Source: CAD feature listing. Evaluate the final solid. Frame: model axes, mm. Give positions to 0.01 mm unless a question says otherwise; leave off trailing zeros. Order: outer loops, then holes, each group sorted by start corner. A loop starts at its lowest first (then second) coordinate and runs counter-clockwise, first axis right, second up. Notation, with made-up numbers: M -27,43 L 4,43 A22 cw 4,53 Z; hole C 30,36 d1. An arc over 180 degrees is marked long. One line per question, with ' | ' between items. Start each with the question number.
from build123d import *

# Parameters (mm, degrees)
SKETCH_7_R           = 35
SKETCH_7_R_2         = 15
EXTRUDE_1_DEPTH      = 15
EXTRUDE_2_REACH      = 817.889
EXTRUDE_2_END_RADIUS = 35
SKETCH_5_R           = 22.5
SKETCH_8_W           = 185.294970715
SKETCH_8_H           = 135.350234673
CUT_EXTRUDE_1_DEPTH  = 25


with BuildPart() as part:
    # 草图7 → 凸台-拉伸1 (new, symmetric)
    with BuildSketch(Plane(origin=(0, 0, 0), x_dir=(1, 0, 0), z_dir=(0, 1, 0))):
        with Locations(Location((0, -500, 0), (0, 0, 270))):
            Circle(SKETCH_7_R)
        with Locations(Location((0, -500, 0), (0, 0, 270))):
            Circle(SKETCH_7_R_2, mode=Mode.SUBTRACT)
    extrude(amount=EXTRUDE_1_DEPTH, both=True)

    # 凸台-拉伸2: up to this cylinder (the profile starts outside it)
    extrude_2_end = Plane(origin=(0, 0, 500), z_dir=(0, -1, 0)) * Cylinder(EXTRUDE_2_END_RADIUS, 1706.778, mode=Mode.PRIVATE)
    # 草图5 → 凸台-拉伸2 (add, up to the surface)
    with BuildSketch(Plane.XY.offset(-280), mode=Mode.PRIVATE) as extrude_2_sk1:
        with Locations(Location((0, 0, 0), (0, 0, 138.189685104))):
            Circle(SKETCH_5_R)
    extrude_2_tool1 = extrude(extrude_2_sk1.sketch, amount=EXTRUDE_2_REACH, mode=Mode.PRIVATE) - extrude_2_end
    add(extrude_2_tool1.solids().sort_by_distance((0, 0, -280))[0])

    # 草图8 → 切除-拉伸1 (cut, symmetric)
    with BuildSketch(Plane(origin=(0, 0, 0), x_dir=(1, 0, 0), z_dir=(0, 1, 0))):
        with Locations((-2.493067274, -527.675117337)):
            Rectangle(SKETCH_8_W, SKETCH_8_H)
    extrude(amount=CUT_EXTRUDE_1_DEPTH, both=True, mode=Mode.SUBTRACT)


solid = part.part
Item 1: Cut plane A-A on z = 29.5. Return the cut outline in (x, y), and give its area (3 significant figures).
Item 2: Line query: line 1 (Y direction, x = -1.5, z = -114.5); line 2 (X direction, y = -2.5, z = 353); line 3 (X direction, y = -0.5, z = -246). Output: solid intervals per line, ascending.
Item 3: Pin query (flat end, axial travel): pin 1 Ø2 at (x, z) = (14, 359.5) entering from -Y; pin 2 Ø1.5 at (y, z) = (13, -181) entering from -X; pin 3 Ø2 at (x, z) = (-16.5, 319.5) entering from -Y. Return the tip coordinate at first contact, or that it passes through.
Results are:
1) outline: C 0,0 d45 | area: 1,590 mm2
2) line 1: y = -22.45 to 22.45 | line 2: x = -22.36 to 22.36 | line 3: x = -22.49 to 22.49
3) pin 1: stops at y = -18.36 | pin 2: stops at x = -18.87 | pin 3: stops at y = -16.31
